Could you check a few things on this model? Use its own coordinates, in mm. Coordinates: 2 decimals unless noted, no trailing zeros. Write each loop counter-clockwise with the first axis right and the second up, starting at its lowest first coordinate (ties: lowest second). Pieces come first, ordered by that corner, then holes.
Item 1: I want a section at D-D on y = 19.05. Please give me the cut outline in (x, z) (3 decimals).
Item 2: If I drill on probe 1 along Y at (x, z) = (93.5, 1.25); probe 2 along Y at (x, z) = (127, 0.5) (3 decimals); probe 3 along X at (y, z) = (171, 0.7), over which ranges is the centre line in solid material (lowest first)?
Item 3: I want a section at A-A on y = 139.7. Please give me the cut outline in (x, z).
Item 4: Thinking about a two-plate mould opening in X: for faces 1 (the cylindrical face through (7.64, 234.06, 1.21)), 2 (the flat face through (53, 122, 2.381)), 3 (the cylindrical face through (129.93, 20.27, 1.17)), which applies, +X half, -X half, draft (parallel to the pull), parting line (faces both ways), or undercut?
Item 5: I want a section at C-C on x = 109.5. Please give me the cut outline in (y, z).
Item 6: For P1, Ø4, axis at x = 127, y = 222.25, coming from the -Z side; P2, Ø1.2, axis at x = 121.5, z = 1.5, coming from the -Y side; P3, Ø0.7, axis at y = 120, z = 1.5, coming from the +X side, each with a flat end and sliding along its axis, tell me the tip position at first contact or that it passes through.
Item 7: I want a section at B-B on z = 0.8. State how many separate pieces and enclosed holes the cut face has, then the cut area to 3 significant figures.
Autodesk Inventor part; units mm, degrees
ref_plane "YZ Plane" through (0, 0, 0) normal (1, 0, 0) x (0, 1, 0)
ref_plane "XZ Plane" through (0, 0, 0) normal (0, 1, 0) x (-1, 0, 0)
ref_plane "XY Plane" through (0, 0, 0) normal (0, 0, 1) x (1, 0, 0)
sketch "Sketch1" plane through (0, 0, 0) normal (0, 0, 1) x (1, 0, 0)
  line L0 (0, 0) -> (139.7, 0)
  line L1 (139.7, 241.3) -> (0, 241.3)
  line L2 (0, 241.3) -> (0, 0)
  line L3 (139.7, 203.2) -> (76.2, 203.2)
  line L4 (76.2, 203.2) -> (76.2, 38.1)
  line L5 (76.2, 38.1) -> (139.7, 38.1)
  line L6 (139.7, 0) -> (139.7, 38.1)
  line L7 (139.7, 203.2) -> (139.7, 241.3)
  circle A0 centre (127, 222.25) radius 3.175
  circle A1 centre (127, 19.05) radius 3.175
  circle A2 centre (19.05, 139.7) radius 4.7625
  circle A3 centre (38.1, 25.4) radius 14.2875
  dimension "d0" = 38.1
  dimension "d1" = 38.1
  dimension "d2" = 241.3
  dimension "d3" = 139.7
  dimension "d4" = 12.7
  dimension "d5" = 12.7
  dimension "d6" = 6.35
  dimension "d7" = 6.35
  dimension "d8" = 19.05
  dimension "d9" = 19.05
  dimension "d10" = 63.5
  dimension "d11" = 9.525
  dimension "d12" = 19.05
  dimension "d13" = 101.6
  dimension "d14" = 28.575
  dimension "d15" = 38.1
  dimension "d16" = 25.4
extrude "Extrusion1" add sketch "Sketch1" along normal blind 2.3813
fillet "Fillet1" radius 25.4 4 edges at (0, 241.3, 1.1906) (139.7, 241.3, 1.1906) (0, 0, 1.1906) (139.7, 0, 1.1906)
properties part number "Plate_VerticalConveyorMotorMount" material "Aluminum-6061"
Response values:
1. outline: (0.807, 0) - (25.301, 0) - (25.301, 2.381) - (0.807, 2.381) - close; (50.899, 0) - (123.825, 0) - (123.825, 2.381) - (50.899, 2.381) - close; (130.175, 0) - (138.893, 0) - (138.893, 2.381) - (130.175, 2.381) - close
2. probe 1: y = 0 to 38.1, 203.2 to 241.3
2. probe 2: y = 3.403 to 15.875, 22.225 to 38.1, 203.2 to 219.075, 225.425 to 237.897
2. probe 3: x = 0 to 76.2
3. outline: (0, 0) - (14.29, 0) - (14.29, 2.38) - (0, 2.38) - close; (23.81, 0) - (76.2, 0) - (76.2, 2.38) - (23.81, 2.38) - close
4. face 1: -X half
4. face 2: draft
4. face 3: undercut
5. outline: (0, 0) - (38.1, 0) - (38.1, 2.38) - (0, 2.38) - close; (203.2, 0) - (241.3, 0) - (241.3, 2.38) - (203.2, 2.38) - close
6. P1: passes through
6. P2: stops at y = 0.87
6. P3: stops at x = 76.2
7. separate pieces: 1
7. enclosed holes: 4
7. area: 21,900 mm2
